```python
from build123d import *

# Parameters (mm, degrees)
EXTRUDE_1_DEPTH          = 20
SKETCH_2_R               = 3
SKETCH_2_R_2             = 1.75
CUT_EXTRUDE_1_DEPTH      = 112
CUT_EXTRUDE_2_DEPTH      = 123
CUT_EXTRUDE_2_DEPTH_BACK = 61
SKETCH_5_W               = 18
SKETCH_5_H               = 40
EXTRUDE_3_DEPTH          = 15
CUT_EXTRUDE_3_DEPTH      = 141.356688476
CUT_EXTRUDE_3_DEPTH_BACK = 141.356688476
SKETCH_6_R               = 2
CUT_EXTRUDE_4_DEPTH      = 141.356688476
CUT_EXTRUDE_4_DEPTH_BACK = 141.356688476
FILLET_1_R               = 6
FILLET_2_R               = 12
CUT_EXTRUDE_5_DEPTH      = 147.372811683
CUT_EXTRUDE_5_DEPTH_BACK = 3
SKETCH_8_W               = 15.6
SKETCH_8_H               = 15.6
SKETCH_9_R               = 3.5
CUT_EXTRUDE_6_DEPTH      = 45


with BuildPart() as part:
    # 草图1 → 凸台-拉伸1 (new, symmetric)
    with BuildSketch(Plane(origin=(0, 0, 0), x_dir=(1, 0, 0), z_dir=(0, 1, 0))):
        Polygon((-18, 0), (0, 0), (0, 90), (-100, 90), (-100, 0), (-82, 0), (-82, 72), (-18, 72), align=None)
    extrude(amount=EXTRUDE_1_DEPTH, both=True)

    # 草图2 → 切除-拉伸1 (cut)
    with BuildSketch(Plane.ZY.offset(100)):
        with Locations((-7, 0)):
            Circle(SKETCH_2_R)
        with Locations((-7, 15.5)):
            Circle(SKETCH_2_R_2)
        with Locations((-7, -15.5)):
            Circle(SKETCH_2_R_2)
    extrude(amount=-CUT_EXTRUDE_1_DEPTH, mode=Mode.SUBTRACT)

    # 草图4 → 切除-拉伸2 (cut, two sides: drawn at the far end of the back side and taken through both)
    with BuildSketch(Plane.ZY.offset(18).offset(-CUT_EXTRUDE_2_DEPTH_BACK)):
        with BuildLine():
            Line((-62, 12.5), (-33, 12.5))
            ThreePointArc((-33, 12.5), (-30.878679656, 11.621320344), (-30, 9.5))
            Line((-30, 9.5), (-30, -9.5))
            ThreePointArc((-30, -9.5), (-30.878679656, -11.621320344), (-33, -12.5))
            Line((-33, -12.5), (-62, -12.5))
            ThreePointArc((-62, -12.5), (-64.121320344, -11.621320344), (-65, -9.5))
            Line((-65, -9.5), (-65, 9.5))
            ThreePointArc((-65, 9.5), (-64.121320344, 11.621320344), (-62, 12.5))
        make_face()
    extrude(amount=CUT_EXTRUDE_2_DEPTH + CUT_EXTRUDE_2_DEPTH_BACK, mode=Mode.SUBTRACT)

    # 草图5 → 凸台-拉伸3 (add)
    with BuildSketch(Plane.XY):
        with Locations((-9, 0)):
            Rectangle(SKETCH_5_W, SKETCH_5_H)
        with Locations((-91, 0)):
            Rectangle(SKETCH_5_W, SKETCH_5_H)
    extrude(amount=EXTRUDE_3_DEPTH)

    # 草图6 → 切除-拉伸3 (cut, two sides: drawn at the far end of the back side and taken through both)
    with BuildSketch(Plane(origin=(0, 20, 0), x_dir=(1, 0, 0), z_dir=(0, 1, 0)).offset(-CUT_EXTRUDE_3_DEPTH_BACK)):
        with Locations(Location((-91, 60, 0), (0, 0, 270))):
            Circle(SKETCH_6_R)
        with Locations(Location((-91, 52, 0), (0, 0, 270))):
            Circle(SKETCH_6_R)
        with Locations(Location((-91, 44, 0), (0, 0, 270))):
            Circle(SKETCH_6_R)
        with Locations(Location((-91, 36, 0), (0, 0, 270))):
            Circle(SKETCH_6_R)
        with Locations(Location((-9, 36, 0), (0, 0, 270))):
            Circle(SKETCH_6_R)
        with Locations(Location((-9, 44, 0), (0, 0, 270))):
            Circle(SKETCH_6_R)
        with Locations(Location((-9, 52, 0), (0, 0, 270))):
            Circle(SKETCH_6_R)
        with Locations(Location((-9, 60, 0), (0, 0, 90))):
            Circle(SKETCH_6_R)
    extrude(amount=CUT_EXTRUDE_3_DEPTH + CUT_EXTRUDE_3_DEPTH_BACK, mode=Mode.SUBTRACT)

    # 草图7 → 切除-拉伸4 (cut, two sides: drawn at the far end of the back side and taken through both)
    with BuildSketch(Plane(origin=(0, 20, 0), x_dir=(1, 0, 0), z_dir=(0, 1, 0)).offset(-CUT_EXTRUDE_4_DEPTH_BACK)):
        with BuildLine():
            Line((-90.5, 85.5), (-63.5, 85.5))
            ThreePointArc((-63.5, 85.5), (-59, 81), (-63.5, 76.5))
            Line((-63.5, 76.5), (-90.5, 76.5))
            ThreePointArc((-90.5, 76.5), (-95, 81), (-90.5, 85.5))
        make_face()
        with BuildLine():
            Line((-9.5, 85.5), (-36.5, 85.5))
            ThreePointArc((-36.5, 85.5), (-41, 81), (-36.5, 76.5))
            Line((-36.5, 76.5), (-9.5, 76.5))
            ThreePointArc((-9.5, 76.5), (-5, 81), (-9.5, 85.5))
        make_face()
    extrude(amount=CUT_EXTRUDE_4_DEPTH + CUT_EXTRUDE_4_DEPTH_BACK, mode=Mode.SUBTRACT)

    # 圆角1
    fillet_1_edges = [part.edges().sort_by_distance(p)[0] for p in [
        (-18, 0, -72),
        (-82, 0, -72),
        (-100, 0, -90),
        (0, 0, -90),
    ]]
    fillet(fillet_1_edges, radius=FILLET_1_R)

    # 圆角2
    fillet_2_edges = [part.edges().sort_by_distance(p)[0] for p in [
        (-9, -20, 15),
        (-9, 20, 15),
        (-91, -20, 15),
        (-91, 20, 15),
    ]]
    fillet(fillet_2_edges, radius=FILLET_2_R)

    # 草图8 → 切除-拉伸5 (cut, two sides: drawn at the far end of the back side and taken through both)
    with BuildSketch(Plane(origin=(0, 0, -90), x_dir=(-1, 0, 0), z_dir=(0, 0, -1)).offset(-CUT_EXTRUDE_5_DEPTH_BACK)):
        with Locations((50, 0)):
            Rectangle(SKETCH_8_W, SKETCH_8_H)
    extrude(amount=CUT_EXTRUDE_5_DEPTH + CUT_EXTRUDE_5_DEPTH_BACK, mode=Mode.SUBTRACT)

    # 草图9 → 切除-拉伸6 (cut, symmetric)
    with BuildSketch(Plane.ZY.offset(50)):
        with Locations((-7, 15.5)):
            Circle(SKETCH_9_R)
        with Locations((-7, -15.5)):
            Circle(SKETCH_9_R)
    extrude(amount=CUT_EXTRUDE_6_DEPTH, both=True, mode=Mode.SUBTRACT)


solid = part.part
```
Here's how the part is built. I have some questions about the finished solid (model axes, mm). A direction names the side the tool comes from. Coordinates: 2 decimals unless noted, no trailing zeros. Order: outer loops, then holes, each group sorted by start corner. A loop starts at its lowest first (then second) coordinate and runs counter-clockwise, first axis right, second up. Notation, with made-up numbers: (-26, 0.5) - (11, 0.5) arc R8 ccw to (11, 7.5) - close; hole circle Ø11 at (85.25, 30.5). An arc over 180 degrees is marked (long way). One line per question, with ' | ' between items. Start each with the question number.
1. If we section it at D-D (z = 8): Write out the boundary of the cut face in (x, y), and give its area (3 significant figures).
2. Please list where these lines run through material, in increasing order: line 1 along Z through (x, y) = (-89, -8); line 2 along X through (y, z) = (18, -52); line 3 along Y through (x, z) = (-96, -7). Write a range as [from, to].
3. If we section it at B-B (z = -81): Write out the boundary of the cut face in (x, y), and give its area (3 significant figures).
4. If we section it at A-A (x = -14.5): Write out the boundary of the cut face in (y, z).
5. I'm going to push flat-ended pins straight in: pin 1 Ø8 at (y, z) = (10, -37) entering from -X; pin 2 Ø3.5 at (x, z) = (-91, -52) entering from +Y; pin 3 Ø10 at (x, y) = (-36.5, -0.5) entering from +Z. Where does each tip first touch, or does it pass through?
6. Which directions (+Z, -Z, +X, -X, +Y, -Y) give clear straight access to the entire face, cutting with the end or side of a thin tool? Please do faces 1 (the flat face through (-23, 0, -76.5)), 2 (the cylindrical face through (-90.87, -11.6, -30.86)), 3 (the flat face through (-100, 0, -24)).
7. If we section it at C-C (x = -28.5): Write out the boundary of the cut face in (y, z).
8. If we mould it in two halves opening along Y, with no side actions, what happens to faces 4 (the cylindrical face through (-8.87, 16.58, 11.39)), 5 (the cylindrical face through (-97.535, -13.765, -7.228)), 6 (the cylindrical face through (-89, -16, -36))? For each: released by +Y, released by -Y, zero draft, split by the parting line, or undercut.
Model answer:
1) outline: (-100, -18.91) - (-82, -18.91) - (-82, 18.91) - (-100, 18.91) - close; (-18, -18.91) - (0, -18.91) - (0, 18.91) - (-18, 18.91) - close | area: 1,360 mm²
2) line 1: z = [-90, -85.5], [-76.5, -65], [-30, 15] | line 2: x = [-100, -93], [-89, -82], [-18, -11], [-7, 0] | line 3: y = [-20, -17.25], [-13.75, -3], [3, 13.75], [17.25, 20]
3) outline: (-100, -20) - (-95, -20) - (-95, 20) - (-100, 20) - close; (-59, -20) - (-41, -20) - (-41, 20) - (-59, 20) - close; (-5, -20) - (0, -20) - (0, 20) - (-5, 20) - close | area: 1,120 mm²
4) outline: (-20, -90) - (20, -90) - (20, -85.5) - (-20, -85.5) - close; (-20, -76.5) - (20, -76.5) - (20, 3) arc R12 ccw to (8, 15) - (-8, 15) arc R12 ccw to (-20, 3) - close; hole circle Ø7 at (-15.5, -7); hole (-12.5, -62) arc R3 ccw to (-9.5, -65) - (9.5, -65) arc R3 ccw to (12.5, -62) - (12.5, -33) arc R3 ccw to (9.5, -30) - (-9.5, -30) arc R3 ccw to (-12.5, -33) - close; hole circle Ø6 at (0, -7); hole circle Ø7 at (15.5, -7)
5) pin 1: stops at x = -100 | pin 2: passes through | pin 3: stops at z = -72
6) face 1: +Y, -Y | face 2: +X, -X | face 3: +Z, -Z, -X, +Y, -Y
7) outline: (-20, -90) - (20, -90) - (20, -85.5) - (-20, -85.5) - close; (-20, -76.5) - (20, -76.5) - (20, -72) - (-20, -72) - close
8) face 4: released by +Y | face 5: undercut | face 6: zero draft
